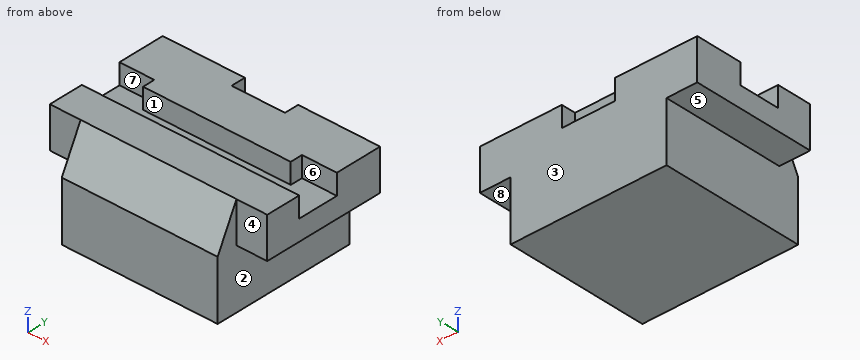
from build123d import *

# Parameters (mm, degrees)
EXTRUDE_1_DEPTH   = 10
EXTRUDE_1_2_DEPTH = 10
EXTRUDE_2_DEPTH   = 10
SKETCH_3_W        = 38
SKETCH_3_H        = 70
EXTRUDE_3_DEPTH   = 9
EXTRUDE_4_DEPTH   = 38
SKETCH_5_W        = 26
SKETCH_5_H        = 7
EXTRUDE_5_DEPTH   = 10
SKETCH_6_W        = 76
SKETCH_6_H        = 70
EXTRUDE_6_DEPTH   = 20


with BuildPart() as part:
    # Sketch 1 → Extrude 1 (new body)
    with BuildSketch(Plane.XY):
        Polygon((-26.5, 23), (-26.5, 1), (9.5, 1), (9.5, 7), (26.5, 7), (26.5, 30), (-13.5, 30), (-13.5, 23), align=None)
    extrude(amount=EXTRUDE_1_DEPTH)



with BuildPart() as body_2:
    # Sketch 1 → Extrude 1 2 (new body)
    with BuildSketch(Plane.XY):
        Polygon((-26.5, -13), (-26.5, -30), (26.5, -30), (26.5, -13), (9.5, -13), align=None)
    extrude(amount=EXTRUDE_1_2_DEPTH)


with BuildPart() as part_1:
    add(part.part)

    add(body_2.part)  # Extrude 2 merges body 2
    # Sketch 2 → Extrude 2 (add)
    with BuildSketch(Plane(origin=(0, 0, 0), x_dir=(-1, 0, 0), z_dir=(0, 0, -1))):
        Polygon((-26.5, -30), (-26.5, 30), (13.5, 30), (13.5, 23), (26.5, 23), (26.5, -30), align=None)
    extrude(amount=EXTRUDE_2_DEPTH)

    # Sketch 3 → Extrude 3 (add)
    with BuildSketch(Plane(origin=(0, 0, -10), x_dir=(-1, 0, 0), z_dir=(0, 0, -1))):
        with Locations((7.5, -5)):
            Rectangle(SKETCH_3_W, SKETCH_3_H)
    extrude(amount=EXTRUDE_3_DEPTH)

    # Sketch 4 → Extrude 4 (add)
    with BuildSketch(Plane(origin=(11.5, 0, 0), x_dir=(0, 0, -1), z_dir=(1, 0, 0))):
        Polygon((10, -40), (-10, -30), (10, -30), align=None)
    extrude(amount=-EXTRUDE_4_DEPTH)

    # Mirror 1: part across plane


with BuildPart() as part_2:
    add(part_1.part)
    add(part_1.part.mirror(Plane(origin=(-26.5, 0, 10), x_dir=(0, 0, 1), z_dir=(-1, 0, 0))))

    # Sketch 5 → Extrude 5 (add)
    with BuildSketch(Plane.XY.offset(-10)):
        with Locations((-26.5, 26.5)):
            Rectangle(SKETCH_5_W, SKETCH_5_H)
    extrude(amount=EXTRUDE_5_DEPTH)

    # Sketch 6 → Extrude 6 (add)
    with BuildSketch(Plane(origin=(0, 0, -19), x_dir=(-1, 0, 0), z_dir=(0, 0, -1))):
        with Locations((26.5, -5)):
            Rectangle(SKETCH_6_W, SKETCH_6_H)
    extrude(amount=EXTRUDE_6_DEPTH)


solid = part_2.part
The listing builds one solid part. Answer for the finished solid, in the listing's coordinates (mm). Face numbers are marked on the shaded views. A direction names the side the tool comes from. Give positions to 0.01 mm unless a question says otherwise; leave off trailing zeros. Loops run counter-clockwise (first coordinate to the right, second up) from the corner with the lowest first, then second, coordinate; pieces in that order, holes last.
Item 1: A cutting plane is placed at C-C (x = -72). Give the vertices of the cut face in (y, z), then the cut area to 3 significant figures.
Derived:
outline: (-30, -10) - (30, -10) - (30, 10) - (7, 10) - (7, 0) - (-13, 0) - (-13, 10) - (-30, 10) - close
area: 1,000 mm2
Item 2: Determine the mould class of the marked faces 1, 2, 3 and 4 for opening direction Y: +Y half, -Y half, draft (parallel to the pull), parting line (faces both ways), or undercut.
Derived:
face 1: undercut
face 2: draft
face 3: +Y half
face 4: -Y half
Item 3: Find the intervals of material crossed by line 1 along X through (y, z) = (8.5, -33); line 2 along Y through (x, z) = (-41, 5.5); line 3 along Z through (x, y) = (-10.5, -2), in increasing order.
Derived:
line 1: x = -64.5 to 11.5
line 2: y = -32.25 to -13, 1 to 30
line 3: z = -39 to 0
Item 4: A cutting plane is placed at D-D (z = -29). Give the vertices of the cut face in (x, y).
Derived:
outline: (-64.5, -40) - (11.5, -40) - (11.5, 30) - (-64.5, 30) - close
Item 5: A tool of negligible diameter and unlimited length cuts with its end or side. For the marked faces 5, 6, 7 and 8, from which of +Z, -Z, +X, -X, +Y, -Y can it reach the whole face along a straight path? Write none if from no direction.
Derived:
face 5: -Z, -X, +Y, -Y
face 6: +Z, +X
face 7: +Z, -X
face 8: -Z, +X, +Y, -Y
Item 6: A cutting plane is placed at A-A (z = 1.5). Give the vertices of the cut face in (x, y), then the cut area to 3 significant figures.
Derived:
outline: (-79.5, -30) - (-64.5, -30) - (-64.5, -34.25) - (11.5, -34.25) - (11.5, -30) - (26.5, -30) - (26.5, -13) - (-79.5, -13) - close; (-79.5, 7) - (-62.5, 7) - (-62.5, 1) - (9.5, 1) - (9.5, 7) - (26.5, 7) - (26.5, 30) - (-13.5, 30) - (-13.5, 23) - (-39.5, 23) - (-39.5, 30) - (-79.5, 30) - close
area: 4,810 mm2
Item 7: Each of these flat-tipped pins is pushed along its axis until it touches: pin 1 Ø1.5 at (y, z) = (10, -30.5) entering from +X; pin 2 Ø3 at (x, z) = (-73, 6) entering from -Y; pin 3 Ø4.5 at (x, y) = (20, 5.5) entering from -Z. Where does it stop, or does it pass through?
Derived:
pin 1: stops at x = 11.5
pin 2: stops at y = -30
pin 3: stops at z = -10
Item 8: A cutting plane is placed at B-B (y = -22). Give the vertices of the cut face in (x, z).
Derived:
outline: (-79.5, -10) - (-64.5, -10) - (-64.5, -39) - (11.5, -39) - (11.5, -10) - (26.5, -10) - (26.5, 10) - (-79.5, 10) - close
